from build123d import *

# Parameters (mm, degrees)
ESQUISSE1_W      = 55.36
ESQUISSE1_H      = 57.1
ESQUISSE1_R      = 1.275
EXTRUSION1_DEPTH = 3
ESQUISSE2_W      = 5
ESQUISSE2_H      = 40
EXTRUSION2_DEPTH = 10
ESQUISSE3_W      = 20
ESQUISSE3_H      = 25
EXTRUSION3_DEPTH = 2
ESQUISSE4_W      = 5
ESQUISSE4_H      = 56.1
EXTRUSION4_DEPTH = 10
ESQUISSE5_W      = 10
ESQUISSE5_H      = 5
EXTRUSION5_DEPTH = 5


with BuildPart() as part:
    # Esquisse1 → Extrusion1 (new body)
    with BuildSketch(Plane(origin=(0, 0, 0), x_dir=(1, 0, 0), z_dir=(0, 1, 0))):
        with Locations((27.68, 28.55)):
            Rectangle(ESQUISSE1_W, ESQUISSE1_H)
        with Locations((9.45, 52.335)):
            Circle(ESQUISSE1_R, mode=Mode.SUBTRACT)
        with Locations((50.36, 52.335)):
            Circle(ESQUISSE1_R, mode=Mode.SUBTRACT)
        with Locations((9.45, 4.765)):
            Circle(ESQUISSE1_R, mode=Mode.SUBTRACT)
        with Locations((50.36, 4.765)):
            Circle(ESQUISSE1_R, mode=Mode.SUBTRACT)
    extrude(amount=EXTRUSION1_DEPTH)

    # Esquisse2 → Extrusion2 (add)
    with BuildSketch(Plane(origin=(0, 3, 0), x_dir=(1, 0, 0), z_dir=(0, 1, 0))):
        with Locations((50.36, 28.55)):
            Rectangle(ESQUISSE2_W, ESQUISSE2_H)
    extrude(amount=EXTRUSION2_DEPTH)

    # Esquisse3 → Extrusion3 (add)
    with BuildSketch(Plane(origin=(0, 3, 0), x_dir=(1, 0, 0), z_dir=(0, 1, 0))):
        with Locations((32.78027682, -0.33040493)):
            Rectangle(ESQUISSE3_W, ESQUISSE3_H)
    extrude(amount=EXTRUSION3_DEPTH)

    # Esquisse4 → Extrusion4 (add)
    with BuildSketch(Plane.XZ):
        with Locations((3, -28.55)):
            Rectangle(ESQUISSE4_W, ESQUISSE4_H)
    extrude(amount=EXTRUSION4_DEPTH)

    # Esquisse5 → Extrusion5 (add)
    with BuildSketch(Plane.XZ):
        with Locations((17.244150354, -57.432970226)):
            Rectangle(ESQUISSE5_W, ESQUISSE5_H)
    extrude(amount=EXTRUSION5_DEPTH)


solid = part.part
Verification items for the finished model (mm, model axes). A direction names the side the tool comes from. Round coordinates to 2 decimals unless told otherwise and drop trailing zeros. Order: outer loops, then holes, each group sorted by start corner. A loop starts at its lowest first (then second) coordinate and runs counter-clockwise, first axis right, second up.
1. Section check A-A on x = 50.36. Record the cut outline in (y, z), then the cut area to 3 significant figures.
Final values:
outline: (0, -57.1) - (3, -57.1) - (3, -53.61) - (0, -53.61) - close; (0, -51.06) - (3, -51.06) - (3, -48.55) - (13, -48.55) - (13, -8.55) - (3, -8.55) - (3, -6.04) - (0, -6.04) - close; (0, -3.49) - (3, -3.49) - (3, 0) - (0, 0) - close
area: 556 mm2
2. Release check for a two-part mould opening along X. For faces 4 (the flat face through (0.5, -5, -29)), 5 (the flat face through (33, 5, 0)), 6 (the cylindrical face through (49.086, 1.479, -4.821)) record: +X half, -X half, draft (parallel to the pull), parting line (faces both ways), or undercut.
Final values:
face 4: -X half
face 5: draft
face 6: undercut
3. Section check D-D on y = 6.5. Record the cut outline in (x, z).
Final values:
outline: (47.86, -48.55) - (52.86, -48.55) - (52.86, -8.55) - (47.86, -8.55) - close
4. Thickness scan on L1, parallel to Z at x = 50.36, y = 0.7; L2, parallel to Y at x = 42.5, z = 6; L3, parallel to Y at x = 21, z = -38.5. Record the ranges inside material, lowest first.
Final values:
L1: z = -57.1 to -53.61, -51.06 to -6.04, -3.49 to 0
L2: y = 3 to 5
L3: y = 0 to 3
5. Access from +Z, -Z, +X, -X, +Y, -Y to the whole of each face (thin tool, end or side, straight path). Record for faces 1 (the flat face through (50, 8, -48.55)), 2 (the flat face through (33, 4, -12.17)), 3 (the flat face through (17, -5, -57)).
Final values:
face 1: -Z, +X, -X, +Y
face 2: -Z, -X, +Y
face 3: +Z, -Z, +X, -Y
6. Go/stop test with flat-tipped pins: P1, Ø5.5, axis at x = 3, y = -6.5, coming from the +Z side; P2, Ø10, axis at x = 10, z = -20, coming from the +Y side; P3, Ø1, axis at y = 7.5, z = -20.5, coming from the -X side. Record where each tip stops, or that it passes through.
Final values:
P1: stops at z = -0.5
P2: stops at y = 3
P3: stops at x = 47.86
7. Section check C-C on z = -13.5. Record the cut outline in (x, y), then the cut area to 3 significant figures.
Final values:
outline: (0, 0) - (0.5, 0) - (0.5, -10) - (5.5, -10) - (5.5, 0) - (55.36, 0) - (55.36, 3) - (52.86, 3) - (52.86, 13) - (47.86, 13) - (47.86, 3) - (0, 3) - close
area: 266 mm2
8. Section check B-B on x = 35.5. Record the cut outline in (y, z).
Final values:
outline: (0, -57.1) - (3, -57.1) - (3, -12.17) - (5, -12.17) - (5, 12.83) - (3, 12.83) - (3, 0) - (0, 0) - close
